```python
from build123d import *
from build123d.topology import SkipClean

# Parameters (mm, degrees)
CROQUIS1_R               = 15.05
CROQUIS1_R_2             = 14.05
SALIENTE_EXTRUIR1_DEPTH  = 0.6
SALIENTE_EXTRUIR2_DEPTH  = 0.4
CROQUIS5_R               = 15.05
CROQUIS5_R_2             = 14.05
SALIENTE_EXTRUIR3_DEPTH  = 0.4
CROQUIS7_R               = 15.05
CROQUIS7_R_2             = 14.05
SALIENTE_EXTRUIR4_DEPTH  = 13
CROQUIS8_W               = 2.286340663
CROQUIS8_H               = 1.122176033
SALIENTE_EXTRUIR5_DEPTH  = 0.6
CROQUIS10_R              = 6.525
CROQUIS10_R_2            = 4.525
SALIENTE_EXTRUIR6_DEPTH  = 1
CROQUIS11_R              = 9.05
CROQUIS11_R_2            = 5.6
SALIENTE_EXTRUIR7_DEPTH  = 5
CROQUIS12_R              = 9.05
CROQUIS12_R_2            = 8.05
SALIENTE_EXTRUIR9_DEPTH  = 1
CROQUIS13_R              = 9.05
CROQUIS13_R_2            = 7.74
SALIENTE_EXTRUIR10_DEPTH = 3.5
CROQUIS14_R              = 8.05
CROQUIS14_R_2            = 6.525
SALIENTE_EXTRUIR11_DEPTH = 1


with BuildPart() as part:
    # Croquis1 → Saliente-Extruir1 (new body)
    with BuildSketch(Plane.XY):
        Circle(CROQUIS1_R)
        Circle(CROQUIS1_R_2, mode=Mode.SUBTRACT)
    extrude(amount=SALIENTE_EXTRUIR1_DEPTH)

    # Croquis2 → Saliente-Extruir2 (add)
    with SkipClean():  # the faces are left unmerged after this step: merging them gives an invalid solid
        with BuildSketch(Plane(origin=(0, 0, 0), x_dir=(-1, 0, 0), z_dir=(0, 0, -1))):
            with BuildLine():
                Line((-2.404789938, 14.856631023), (-2.404789938, 13.842669011))
                ThreePointArc((-2.404789938, 13.842669011), (0, 14.05), (2.404789938, 13.842669011))
                Line((2.404789938, 13.842669011), (2.404789938, 14.856631023))
                ThreePointArc((2.404789938, 14.856631023), (0, 15.05), (-2.404789938, 14.856631023))
            make_face()
            with BuildLine():
                Line((14.856631023, 2.404789938), (13.842669011, 2.404789938))
                ThreePointArc((13.842669011, 2.404789938), (14.05, 0), (13.842669011, -2.404789938))
                Line((13.842669011, -2.404789938), (14.856631023, -2.404789938))
                ThreePointArc((14.856631023, -2.404789938), (15.05, 0), (14.856631023, 2.404789938))
            make_face()
            with BuildLine():
                Line((2.404789938, -14.856631023), (2.404789938, -13.842669011))
                ThreePointArc((2.404789938, -13.842669011), (0, -14.05), (-2.404789938, -13.842669011))
                Line((-2.404789938, -13.842669011), (-2.404789938, -14.856631023))
                ThreePointArc((-2.404789938, -14.856631023), (0, -15.05), (2.404789938, -14.856631023))
            make_face()
            with BuildLine():
                Line((-14.856631023, -2.404789938), (-13.842669011, -2.404789938))
                ThreePointArc((-13.842669011, -2.404789938), (-14.05, 0), (-13.842669011, 2.404789938))
                Line((-13.842669011, 2.404789938), (-14.856631023, 2.404789938))
                ThreePointArc((-14.856631023, 2.404789938), (-15.05, 0), (-14.856631023, -2.404789938))
            make_face()
        extrude(amount=SALIENTE_EXTRUIR2_DEPTH)

    # Croquis4 → Revolución1 (revolve)
    with SkipClean():  # the faces are left unmerged after this step: merging them gives an invalid solid
        with BuildSketch(Plane(origin=(0, 0, 0), x_dir=(0, 0, -1), z_dir=(1, 0, 0)), mode=Mode.PRIVATE) as revoluci_n1_sk:
            Polygon((-0.6, 15.05), (-4.6, 9.05), (-4.6, 8.05), (-0.6, 14.05), align=None)
        revolve(revoluci_n1_sk.sketch.rotate(Axis((0, 0, 0), (0, 0, 1)), 80.14476262), axis=Axis((0, 0, 0), (0, 0, 1)))

    # Croquis5 → Saliente-Extruir3 (add)
    with SkipClean():  # the faces are left unmerged after this step: merging them gives an invalid solid
        with BuildSketch(Plane(origin=(0, 0, 0), x_dir=(-1, 0, 0), z_dir=(0, 0, -1))):
            Circle(CROQUIS5_R)
            Circle(CROQUIS5_R_2, mode=Mode.SUBTRACT)
        extrude(amount=SALIENTE_EXTRUIR3_DEPTH)

    # Croquis7 → Saliente-Extruir4 (add)
    with SkipClean():  # the faces are left unmerged after this step: merging them gives an invalid solid
        with BuildSketch(Plane(origin=(0, 0, -0.4), x_dir=(-1, 0, 0), z_dir=(0, 0, -1))):
            Circle(CROQUIS7_R)
            Circle(CROQUIS7_R_2, mode=Mode.SUBTRACT)
        extrude(amount=SALIENTE_EXTRUIR4_DEPTH)

    # Croquis8 → Saliente-Extruir5 (add)
    with SkipClean():  # the faces are left unmerged after this step: merging them gives an invalid solid
        with BuildSketch(Plane(origin=(0, 0, -13.4), x_dir=(-1, 0, 0), z_dir=(0, 0, -1))):
            with Locations((-0.064707754, 15.075419169)):
                Rectangle(CROQUIS8_W, CROQUIS8_H)
        extrude(amount=-SALIENTE_EXTRUIR5_DEPTH)



with BuildPart() as body_2:
    # Croquis10 → Saliente-Extruir6 (new body)
    with BuildSketch(Plane.XY.offset(4.6)):
        Circle(CROQUIS10_R)
        Circle(CROQUIS10_R_2, mode=Mode.SUBTRACT)
    extrude(amount=SALIENTE_EXTRUIR6_DEPTH)

    # Croquis11 → Saliente-Extruir7 (add)
    with BuildSketch(Plane.XY.offset(5.6)):
        Circle(CROQUIS11_R)
        Circle(CROQUIS11_R_2, mode=Mode.SUBTRACT)
    extrude(amount=SALIENTE_EXTRUIR7_DEPTH)


with BuildPart() as part_1:
    with SkipClean():  # the faces are left unmerged after this step: merging them gives an invalid solid
        add(part.part)

        add(body_2.part)  # Saliente-Extruir9 merges body 2
        # Croquis12 → Saliente-Extruir9 (add)
        with BuildSketch(Plane.XY.offset(4.6)):
            Circle(CROQUIS12_R)
            with Locations(Location((0, 0, 0), (0, 0, 90))):
                Circle(CROQUIS12_R_2, mode=Mode.SUBTRACT)
        extrude(amount=SALIENTE_EXTRUIR9_DEPTH)

    # Croquis13 → Saliente-Extruir10 (add)
    with SkipClean():  # the faces are left unmerged after this step: merging them gives an invalid solid
        with BuildSketch(Plane.XY.offset(10.6)):
            Circle(CROQUIS13_R)
            Circle(CROQUIS13_R_2, mode=Mode.SUBTRACT)
        extrude(amount=SALIENTE_EXTRUIR10_DEPTH)

    # Croquis14 → Saliente-Extruir11 (add)
    with SkipClean():  # the faces are left unmerged after this step: merging them gives an invalid solid
        with BuildSketch(Plane(origin=(0, 0, 4.6), x_dir=(-1, 0, 0), z_dir=(0, 0, -1))):
            Circle(CROQUIS14_R)
            Circle(CROQUIS14_R_2, mode=Mode.SUBTRACT)
        extrude(amount=-SALIENTE_EXTRUIR11_DEPTH)


solid = part_1.part
```
For this review, take the finished solid that the model builds, in its own axes (mm). A direction names the side the tool comes from. Give positions to 0.01 mm unless a question says otherwise; leave off trailing zeros. Order: outer loops, then holes, each group sorted by start corner. A loop starts at its lowest first (then second) coordinate and runs counter-clockwise, first axis right, second up.
1) Take a section at C-C (z = -3.75). Give the boundary of the cut face in (x, y), then the cut area to 3 significant figures.
2) Insertion check: pin 1 (1.5 mm diameter, centred on x = 8.5, z = 8, fed in from +Y); pin 2 (2 mm diameter, centred on x = 4, y = 12, fed in from +Z); pin 3 (1 mm diameter, centred on x = 5.5, y = -8, fed in from +Z); pin 4 (5.5 mm diameter, centred on x = 0, y = 0, fed in from +Z). Each pin has a flat end and moves straight along its axis. Give the tip position at first contact, or say it passes through.
3) For faces 4 (the face through (3.572, -6.867, 12.326)), 5 (the face through (4.316, 1.359, 5.093)), list the 3-axis set-ups (+Z, -Z, +X, -X, +Y, -Y) from which the entire face can be reached by the end or side of a thin tool; tool diameter is ignored.
4) Take a section at B-B (z = 11.5). Give the boundary of the cut face in (x, y).
5) The part is to be moulded in two halves that separate along Y. For faces 1 (the face through (3, 5, 10.6)), 2 (the face through (-8, 12, -13.4)), 3 (the face through (3.556, 8.638, 4.406)), say which applies: released by +Y, released by -Y, zero draft, split by the parting line, or undercut.
6) Wall thickness on line 1 (Y direction, x = 0, z = 7.65); line 2 (Y direction, x = 0, z = 0.2); line 3 (X direction, y = 11, z = -2.75): over which ranges is each line inside the solid? List them lowest first.
Derived:
1. outline: circle Ø30.1 at (0, 0); hole circle Ø28.1 at (0, 0)
1. area: 91.4 mm2
2. pin 1: stops at y = 4.67
2. pin 2: stops at z = 2.87
2. pin 3: stops at z = 4.49
2. pin 4: passes through
3. face 4: +Z
3. face 5: +Z, -Z
4. outline: circle Ø18.1 at (0, 0); hole circle Ø15.48 at (0, 0)
5. face 1: undercut
5. face 2: zero draft
5. face 3: split by the parting line
6. line 1: y = -9.05 to -5.6, 5.6 to 9.05
6. line 2: y = -15.05 to -14.05, 14.05 to 15.05
6. line 3: x = -10.27 to -8.74, 8.74 to 10.27
